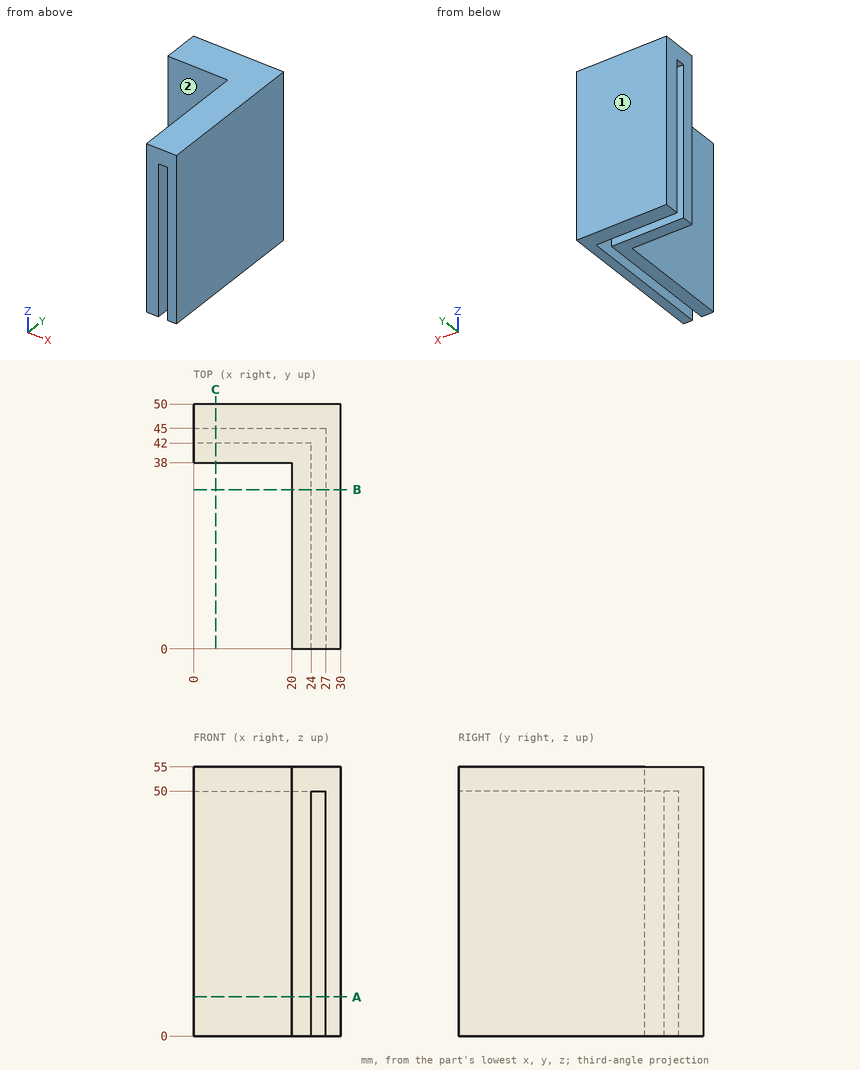
The drawing under review shows one solid part. Ordinate dimensions are in mm from its lowest x, y, z. A direction names the side the tool comes from. Coordinates: 2 decimals unless noted, no trailing zeros. Loops run counter-clockwise (first coordinate to the right, second up) from the corner with the lowest first, then second, coordinate; pieces in that order, holes last.
Item 1: For the marked faces 1 and 2, list the 3-axis set-ups (+Z, -Z, +X, -X, +Y, -Y) from which the entire face can be reached by the end or side of a thin tool; tool diameter is ignored.
Completed:
face 1: +Z, -Z, +X, -X, +Y
face 2: +Z, -Z, -X, -Y
Item 2: Add section C-C (x = 4.5). Write out the cut boundary in (y, z).
Completed:
outline: (38, 0) - (42, 0) - (42, 50) - (45, 50) - (45, 0) - (50, 0) - (50, 55) - (38, 55) - close
Item 3: Wall thickness on L1, parallel to Y at x = 23.25, z = 32.5; L2, parallel to X at y = 32, z = 38; L3, parallel to Y at x = 10.75, z = 7: over which ranges is each line inside the solid? List them lowest first.
Completed:
L1: y = 0 to 42, 45 to 50
L2: x = 20 to 24, 27 to 30
L3: y = 38 to 42, 45 to 50
Item 4: Clearance check with flat-ended pins moving along their axes: pin 1 (1 mm diameter, centred on y = 34.5, z = 27, fed in from -X); pin 2 (13.5 mm diameter, centred on x = 10.5, z = 31.5, fed in from -Y). State where each tip first meets the part, or that it passes through.
Completed:
pin 1: stops at x = 20
pin 2: stops at y = 38
Item 5: Add section B-B (y = 32.5). Write out the cut boundary in (x, z).
Completed:
outline: (20, 0) - (24, 0) - (24, 50) - (27, 50) - (27, 0) - (30, 0) - (30, 55) - (20, 55) - close
Item 6: Add section A-A (z = 8). Write out the cut boundary in (x, y).
Completed:
outline: (0, 38) - (20, 38) - (20, 0) - (24, 0) - (24, 42) - (0, 42) - close; (0, 45) - (27, 45) - (27, 0) - (30, 0) - (30, 50) - (0, 50) - close
